```python
from build123d import *

# Parameters (mm, degrees)
BASES_R                     = 6.35
BASE_DEPTH                  = 5.4
TOPBORES_R                  = 1.4
TOP_BORE_DEPTH              = 11.478788098
HORN_HALF_DEPTH             = 2.5
HORNATTACHS_R               = 0.5
HORN_ATTACH_DEPTH           = 21.913031822
HA_LP_COUNT                 = 4
HA_LP_PITCH                 = 3
HORN_BODIES_COPY_1_SKETCH_R = 0.5
HORN_BODIES_COPY_1_DEPTH    = 21.913031822
HORN_BODIES_COPY_2_SKETCH_R = 0.5
HORN_BODIES_COPY_2_DEPTH    = 21.913031822
HORN_BODIES_COPY_3_SKETCH_R = 0.5
HORN_BODIES_COPY_3_DEPTH    = 21.913031822
TOOTH_DEPTH                 = 3
TOOTH_CP_COUNT              = 26
BOTTOMBORES_R               = 2.6
BOTTOM_BORE_DEPTH           = 3
HOLDINGSHAFTS_R             = 6.35
HOLDINGSHAFTS_R_2           = 4.25
HOLDING_SHAFT_DEPTH         = 2.9
RIB_DEPTH                   = 0.5
RIB_CP_COUNT                = 4
TOPCUTS_R                   = 4.375
TOP_CUT_DEPTH               = 1
TOPPOCKETCYLINDERS_R        = 3.375
TOPPOCKETCYLINDERS_R_2      = 2.875
TOP_POCKET_CYLINDER_DEPTH   = 1.35


with BuildPart() as part:
    # BaseS → BASE (new body)
    with BuildSketch(Plane(origin=(0, 0, 0), x_dir=(1, 0, 0), z_dir=(0, 1, 0))):
        with Locations(Location((0, 0, 0), (0, 0, 90))):
            Circle(BASES_R)
    extrude(amount=BASE_DEPTH)

    # TopBoreS → TOP BORE (cut, through all)
    with BuildSketch(Plane(origin=(0, 5.4, 0), x_dir=(1, 0, 0), z_dir=(0, 1, 0))):
        with Locations(Location((0, 0, 0), (0, 0, 270))):
            Circle(TOPBORES_R)
    extrude(amount=-TOP_BORE_DEPTH, mode=Mode.SUBTRACT)

    # HornHalfS → HORN HALF (add)
    with BuildSketch(Plane(origin=(0, 5.4, 0), x_dir=(1, 0, 0), z_dir=(0, 1, 0))):
        with BuildLine():
            Line((-2.609740545, 16.990167671), (-4.891612682, 4.049027706))
            ThreePointArc((-4.891612682, 4.049027706), (0, 6.35), (4.891612682, 4.049027706))
            Line((4.891612682, 4.049027706), (2.609740545, 16.990167671))
            ThreePointArc((2.609740545, 16.990167671), (0, 19.18), (-2.609740545, 16.990167671))
        make_face()
    horn_half = extrude(amount=-HORN_HALF_DEPTH)

    # HornAttachS → HORN ATTACH (cut, through all)
    with BuildSketch(Plane(origin=(0, 5.4, 0), x_dir=(1, 0, 0), z_dir=(0, 1, 0))):
        with Locations(Location((0, 16.53, 0), (0, 0, 270))):
            Circle(HORNATTACHS_R)
    horn_attach = extrude(amount=-HORN_ATTACH_DEPTH, mode=Mode.SUBTRACT)

    # HA LP: HORN ATTACH ×4
    with Locations(*[(0, 0, i * HA_LP_PITCH) for i in range(1, HA_LP_COUNT)]):
        add(horn_attach, mode=Mode.SUBTRACT)

    # HORN BODIES: HORN HALF, HORN ATTACH across plane
    add(horn_half.mirror(Plane.XY))
    add(horn_attach.mirror(Plane.XY), mode=Mode.SUBTRACT)

    # HORN BODIES copy 1 sketch → HORN BODIES copy 1 (cut, through all)
    with BuildSketch(Plane(origin=(0, 5.4, -3), x_dir=(1, 0, 0), z_dir=(0, 1, 0))):
        with Locations((0, -16.53)):
            Circle(HORN_BODIES_COPY_1_SKETCH_R)
    extrude(amount=-HORN_BODIES_COPY_1_DEPTH, mode=Mode.SUBTRACT)

    # HORN BODIES copy 2 sketch → HORN BODIES copy 2 (cut, through all)
    with BuildSketch(Plane(origin=(0, 5.4, -6), x_dir=(1, 0, 0), z_dir=(0, 1, 0))):
        with Locations((0, -16.53)):
            Circle(HORN_BODIES_COPY_2_SKETCH_R)
    extrude(amount=-HORN_BODIES_COPY_2_DEPTH, mode=Mode.SUBTRACT)

    # HORN BODIES copy 3 sketch → HORN BODIES copy 3 (cut, through all)
    with BuildSketch(Plane(origin=(0, 5.4, -9), x_dir=(1, 0, 0), z_dir=(0, 1, 0))):
        with Locations((0, -16.53)):
            Circle(HORN_BODIES_COPY_3_SKETCH_R)
    extrude(amount=-HORN_BODIES_COPY_3_DEPTH, mode=Mode.SUBTRACT)

    # ToothS → TOOTH (cut)
    with BuildSketch(Plane.XZ):
        with BuildLine():
            Line((0, -2.9), (0.262912611, -2.586672952))
            ThreePointArc((0.262912611, -2.586672952), (0, -2.6), (-0.262912611, -2.586672952))
            Line((-0.262912611, -2.586672952), (0, -2.9))
        make_face()
    tooth = extrude(amount=-TOOTH_DEPTH, mode=Mode.SUBTRACT)

    # TOOTH CP: TOOTH ×26 about axis
    tooth_cp_axis = Axis((0, 0, 0), (0, 1, 0))
    for i in range(1, TOOTH_CP_COUNT):
        add(tooth.rotate(tooth_cp_axis, i * 360 / TOOTH_CP_COUNT), mode=Mode.SUBTRACT)

    # BottomBoreS → BOTTOM BORE (cut)
    with BuildSketch(Plane(origin=(0, 0, 0), x_dir=(-1, 0, 0), z_dir=(0, -1, 0))):
        Circle(BOTTOMBORES_R)
    extrude(amount=-BOTTOM_BORE_DEPTH, mode=Mode.SUBTRACT)

    # HoldingShaftS → HOLDING SHAFT (cut)
    with BuildSketch(Plane.XZ):
        Circle(HOLDINGSHAFTS_R)
        with Locations(Location((0, 0, 0), (0, 0, 270))):
            Circle(HOLDINGSHAFTS_R_2, mode=Mode.SUBTRACT)
    extrude(amount=-HOLDING_SHAFT_DEPTH, mode=Mode.SUBTRACT)

    # RibS → RIB (add, symmetric)
    with BuildSketch(Plane.XY):
        Polygon((4.21, 1), (5.804289299, 2.9), (4.21, 2.9), (4.16, 2.9), (4.16, 1), align=None)
    rib = extrude(amount=RIB_DEPTH, both=True)

    # RIB CP: RIB ×4 about axis
    rib_cp_axis = Axis((0, 0, 0), (0, 1, 0))
    for i in range(1, RIB_CP_COUNT):
        add(rib.rotate(rib_cp_axis, i * 360 / RIB_CP_COUNT))

    # TopCutS → TOP CUT (cut)
    with BuildSketch(Plane(origin=(0, 5.4, 0), x_dir=(1, 0, 0), z_dir=(0, 1, 0))):
        with Locations(Location((0, 0, 0), (0, 0, 270))):
            Circle(TOPCUTS_R)
    extrude(amount=-TOP_CUT_DEPTH, mode=Mode.SUBTRACT)

    # TopPocketCylinderS → TOP POCKET CYLINDER (add)
    with BuildSketch(Plane(origin=(0, 4.4, 0), x_dir=(1, 0, 0), z_dir=(0, 1, 0))):
        with Locations(Location((0, 0, 0), (0, 0, 270))):
            Circle(TOPPOCKETCYLINDERS_R)
        with Locations(Location((0, 0, 0), (0, 0, 270))):
            Circle(TOPPOCKETCYLINDERS_R_2, mode=Mode.SUBTRACT)
    extrude(amount=TOP_POCKET_CYLINDER_DEPTH)


solid = part.part
```
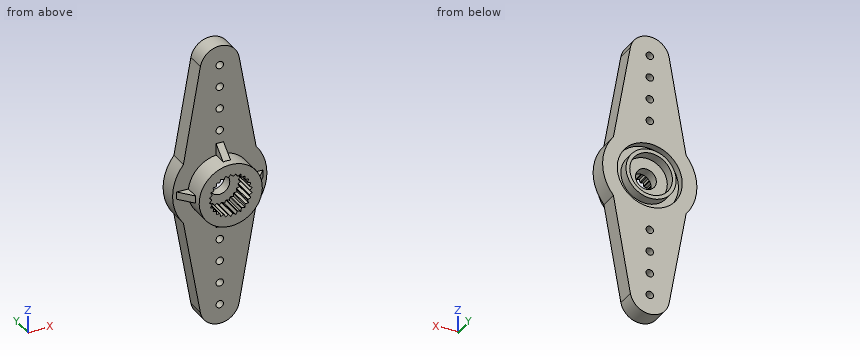
Work out the finished part from the listing and answer in its coordinate system (mm). Coordinates: 2 decimals unless noted, no trailing zeros. Write each loop counter-clockwise with the first axis right and the second up, starting at its lowest first coordinate (ties: lowest second). Pieces come first, ordered by that corner, then holes. Notation, with made-up numbers: (-26.75, 39) - (23.25, 39) arc R14 ccw to (23.25, 49) - close; hole circle Ø10 at (31, 67.25). An arc over 180 degrees is marked (long way). Answer as a JSON object with one key per item and string values.
Q1. Consider L1, parallel to X at y = 4.75, z = 0 (3 decimals); L2, parallel to X at y = 3.65, z = 0; L3, parallel to Y at x = 1, z = -14.5. Determine where each line is inside the solid, lowest interval first. Write a range as from..to.
Results list:
{"L1": "x = -6.35..-4.375, -3.375..-2.875, 2.875..3.375, 4.375..6.35", "L2": "x = -6.35..-1.4, 1.4..6.35", "L3": "y = 2.9..5.4"}
Q2. Find section C-C (z = -16.5). Write down the section's boundary in (x, y).
Results list:
{"outline": "(-2.7, 2.9) - (-0.5, 2.9) - (-0.5, 5.4) - (-2.7, 5.4) - close; (0.5, 2.9) - (2.7, 2.9) - (2.7, 5.4) - (0.5, 5.4) - close"}
Q3. Given pin 1 Ø0.5 at (y, z) = (2, -5) entering from +X; pin 2 Ø0.8 at (x, y) = (5.5, 2) entering from -Z; pin 3 Ø6.5 at (x, z) = (-1, 9) entering from +Y; pin 4 Ø0.8 at (y, z) = (1.5, 5.5) entering from -X, each flat-ended and moving along its own axis, determine where each tip first touches the part or whether it passes through.
Results list:
{"pin 1": "stops at x = 0.5", "pin 2": "stops at z = -0.5", "pin 3": "stops at y = 5.4", "pin 4": "passes through"}
Q4. Find section D-D (z = -9). Write down the section's boundary in (x, y).
Results list:
{"outline": "(-4.02, 2.9) - (4.02, 2.9) - (4.02, 5.4) - (-4.02, 5.4) - close"}
Q5. Find section A-A (y = 4). State how many separate pieces and enclosed holes the cut face has, plus the area to 3 significant figures.
Results list:
{"separate pieces": "1", "enclosed holes": "9", "area": "294 mm^2"}
Q6. Find section B-B (z = 16.53). Write down the section's boundary in (x, y), plus the area to 3 significant figures.
Results list:
{"outline": "(-2.69, 2.9) - (-0.5, 2.9) - (-0.5, 5.4) - (-2.69, 5.4) - close; (0.5, 2.9) - (2.69, 2.9) - (2.69, 5.4) - (0.5, 5.4) - close", "area": "11.0 mm^2"}
